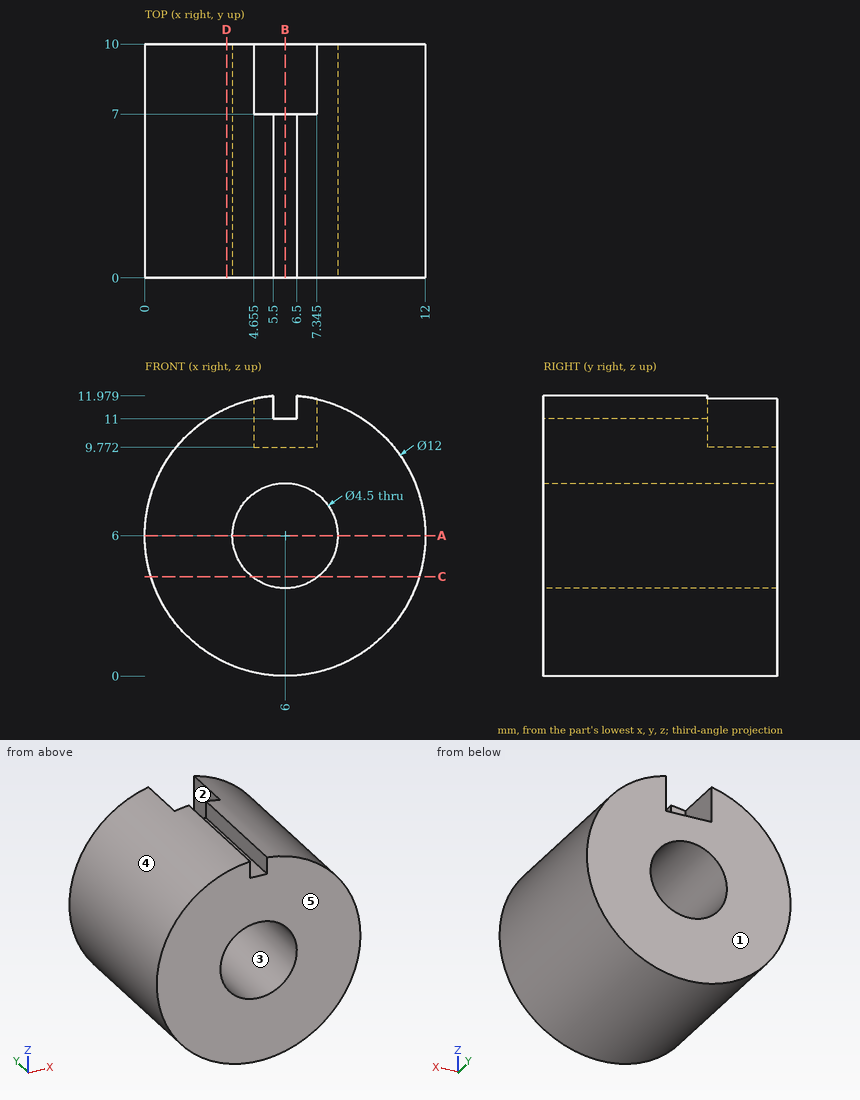
Answer from the drawing. Dimensions are ordinates in mm from the lowest x, y and z of the part. A direction names the side the tool comes from. Round coordinates to 2 decimals unless told otherwise and drop trailing zeros. Loops run counter-clockwise (first coordinate to the right, second up) from the corner with the lowest first, then second, coordinate; pieces in that order, holes last.
Q1. Each of these flat-tipped pins is pushed along its axis until it touches: pin 1 (0.8 mm diameter, centred on y = 3.5, z = 11.5, fed in from +X); pin 2 (3 mm diameter, centred on x = 1.5, y = 8.5, fed in from +Z) (1 decimal); pin 3 (1.3 mm diameter, centred on x = 6, y = 8.5, fed in from +Z); pin 4 (3.5 mm diameter, centred on x = 6, z = 6, fed in from -Y). Where does it stop, or does it pass through?
Q2. Section B-B on x = 6 is taken. Write down the section's boundary in (y, z).
Q3. Section A-A on z = 6 is taken. Write down the section's boundary in (x, y).
Q4. Determine the mould class of the marked faces 3, 4 and 5 for opening direction X: released by +X, released by -X, zero draft, split by the parting line, or undercut.
Q5. Consider probe 1 along X at (y, z) = (7, 6); probe 2 along Z at (x, y) = (6.5, 7.75) (1 decimal); probe 3 along X at (y, z) = (5, 5.25). Determine where each line is inside the solid, lowest interval first.
Q6. Section D-D on x = 3.5 is taken. Write down the section's boundary in (y, z) (1 decimal).
Q7. Section C-C on z = 4.25 is taken. Write down the section's boundary in (x, y) (1 decimal).
Q8. Which of the six approach directions +Z, -Z, +X, -X, +Y, -Y give full straight-line access (tool end or side, diameter ignored) to the marked faces 1 and 2?
Output:
1. pin 1: stops at x = 9.16
1. pin 2: stops at z = 11.2
1. pin 3: stops at z = 9.77
1. pin 4: passes through
2. outline: (0, 0) - (10, 0) - (10, 3.75) - (0, 3.75) - close; (0, 8.25) - (10, 8.25) - (10, 9.77) - (7, 9.77) - (7, 11) - (0, 11) - close
3. outline: (0, 0) - (3.75, 0) - (3.75, 10) - (0, 10) - close; (8.25, 0) - (12, 0) - (12, 10) - (8.25, 10) - close
4. face 3: undercut
4. face 4: split by the parting line
4. face 5: zero draft
5. probe 1: x = 0 to 3.75, 8.25 to 12
5. probe 2: z = 0 to 3.8, 8.2 to 9.8
5. probe 3: x = 0.05 to 3.88, 8.12 to 11.95
6. outline: (0, 0.5) - (10, 0.5) - (10, 11.5) - (0, 11.5) - close
7. outline: (0.3, 0) - (4.6, 0) - (4.6, 10) - (0.3, 10) - close; (7.4, 0) - (11.7, 0) - (11.7, 10) - (7.4, 10) - close
8. face 1: +Z, -Z, +X, -X, +Y
8. face 2: +Z, +Y
